Source: CAD feature listing. Evaluate the final solid. Frame: model axes, mm. Coordinates: 2 decimals unless noted, no trailing zeros. Write each loop counter-clockwise with the first axis right and the second up, starting at its lowest first coordinate (ties: lowest second). Pieces come first, ordered by that corner, then holes. Notation, with made-up numbers: M 24,85.25 L 58,85.25 A22 ccw 58,101.25 Z; hole C 82.5,14.25 d9. An arc over 180 degrees is marked long. Write item = value, one per line. Start each with the question number.
1. Section query B-B (z = -161). Output: boundary loops of the cut face in (x, y), then the cut area to 3 significant figures.
2. Section query A-A (y = 1.7). Give the number of separate pieces and of enclosed holes in the cut face, then the cut area to 3 significant figures.
3. Line query: line 1 along Y through (x, z) = (6.75, -183); line 2 along X through (y, z) = (1.4, -136.5). Output: solid intervals per line, ascending.
4. Pull-direction query (Z, two-part tool) for faces 1 (the face through (0, 0, -4)), 2 (the face through (0, 1, -4)); classes: pulls with the +Z half, pulls with the -Z half, needs draft (parallel to the pull), parting line crosses it, or undercut.
5. Pin query (flat end, axial travel): pin 1 Ø0.6 at (x, y) = (-1, 2) entering from +Z; pin 2 Ø1 at (x, z) = (4, 51.5) entering from +Y; pin 3 Ø1.6 at (y, z) = (2, 41.5) entering from +X. Return the tip coordinate at first contact, or that it passes through.
```python
from build123d import *

# Parameters (mm, degrees)
ESQUISSE1_W                    = 20
ESQUISSE1_H                    = 500
BOSS_EXTRU_1_DEPTH             = 1
ESQUISSE2_W                    = 7
ESQUISSE2_H                    = 7
BOSS_EXTRU_2_DEPTH             = 2
R_P_TITION_LIN_AIRE1_COUNT     = 7
R_P_TITION_LIN_AIRE1_PITCH     = 30
R_P_TITION_LIN_AIRE1_COL_COUNT = 9
R_P_TITION_LIN_AIRE1_COL_PITCH = 30


with BuildPart() as part:
    # Esquisse1 → Boss.-Extru.1 (new body)
    with BuildSketch(Plane(origin=(0, 0, 0), x_dir=(1, 0, 0), z_dir=(0, 1, 0))):
        Rectangle(ESQUISSE1_W, ESQUISSE1_H)
    extrude(amount=BOSS_EXTRU_1_DEPTH)

    # Esquisse2 → Boss.-Extru.2 (add)
    with BuildSketch(Plane(origin=(0, 1, 0), x_dir=(1, 0, 0), z_dir=(0, 1, 0))):
        with Locations((0, 19.127958594)):
            Rectangle(ESQUISSE2_W, ESQUISSE2_H)
    boss_extru_2 = extrude(amount=BOSS_EXTRU_2_DEPTH)

    # Répétition linéaire1: Boss.-Extru.2 ×7
    with Locations(*[(0, 0, -i * R_P_TITION_LIN_AIRE1_PITCH) for i in range(1, R_P_TITION_LIN_AIRE1_COUNT)]):
        add(boss_extru_2)

    # Répétition linéaire1 col: Boss.-Extru.2 ×9
    with Locations(*[(0, 0, i * R_P_TITION_LIN_AIRE1_COL_PITCH) for i in range(1, R_P_TITION_LIN_AIRE1_COL_COUNT)]):
        add(boss_extru_2)


solid = part.part
```
Results are:
q1.outline = M -10,0 L 10,0 L 10,1 L -10,1 Z
q1.area = 20.0 mm^2
q2.separate_pieces = 15
q2.enclosed_holes = 0
q2.area = 735 mm^2
q3.line_1 = 0 to 1
q3.line_2 = -3.5 to 3.5
q4.face_1 = needs draft
q4.face_2 = undercut
q5.pin_1 = 224.37
q5.pin_2 = 1
q5.pin_3 = 3.5
